Build history of the part. All positions in model axes, mm. A direction names the side the tool comes from. Round coordinates to 2 decimals unless told otherwise and drop trailing zeros. Loops run counter-clockwise (first coordinate to the right, second up) from the corner with the lowest first, then second, coordinate; pieces in that order, holes last. Notation, with made-up numbers: (-16, -20) -> (-4, -20) arc R21 ccw to (-4, -13) -> close; hole circle Ø7 at (20, 81). An arc over 180 degrees is marked (long way). Put each result on its own line as item: value. Start each with the question number.
```python
from build123d import *

# Parameters (mm, degrees)
SKETCH1_R           = 36.125
BOSS_EXTRUDE1_DEPTH = 12
SKETCH3_R           = 37.625
BOSS_EXTRUDE3_DEPTH = 1.5
SKETCH4_R           = 37.625
BOSS_EXTRUDE4_DEPTH = 1.5
SKETCH5_R           = 28
BOSS_EXTRUDE5_DEPTH = 10
SKETCH6_R           = 12.5
CUT_EXTRUDE1_DEPTH  = 25


with BuildPart() as part:
    # Sketch1 → Boss-Extrude1 (new body)
    with BuildSketch(Plane(origin=(0, 0, 0), x_dir=(1, 0, 0), z_dir=(0, 1, 0))):
        Circle(SKETCH1_R)
    extrude(amount=BOSS_EXTRUDE1_DEPTH)

    # Sketch3 → Boss-Extrude3 (add)
    with BuildSketch(Plane(origin=(0, 12, 0), x_dir=(1, 0, 0), z_dir=(0, 1, 0))):
        Circle(SKETCH3_R)
    extrude(amount=BOSS_EXTRUDE3_DEPTH)

    # Sketch4 → Boss-Extrude4 (add)
    with BuildSketch(Plane.XZ):
        Circle(SKETCH4_R)
    extrude(amount=BOSS_EXTRUDE4_DEPTH)

    # Sketch5 → Boss-Extrude5 (add)
    with BuildSketch(Plane.XZ.offset(1.5)):
        Circle(SKETCH5_R)
    extrude(amount=BOSS_EXTRUDE5_DEPTH)

    # Sketch6 → Cut-Extrude1 (cut)
    with BuildSketch(Plane(origin=(0, 13.5, 0), x_dir=(1, 0, 0), z_dir=(0, 1, 0))):
        Circle(SKETCH6_R)
    extrude(amount=-CUT_EXTRUDE1_DEPTH, mode=Mode.SUBTRACT)


solid = part.part
```
Item 1: 3-axis set-ups, long thin cutter, end or side, ignore diameter. For faces 4 (the face through (6, -11.5, -12)), 5 (the face through (-28, -1.5, -3)), 6 (the face through (-34, 0, 14)): which of +Z, -Z, +X, -X, +Y, -Y reach the whole face in a straight line?
Item 2: Cut at B-B on x = 0. Write the cut outline in (y, z) (3 decimals).
Item 3: Pull direction Y, two halves, no side cores. Call faces 1 (the face through (19.42, 5.92, -30.46)), 2 (the face through (-9, 13.5, -9)), 3 (the face through (-27.73, 12.74, -25.43)): +Y half, -Y half, draft (parallel to the pull), parting line (faces both ways), or undercut.
Item 4: Cut at D-D on y = -5.25. Write the cut outline in (x, z), then the cut area to 3 significant figures.
Item 5: Drop flat-ended pins along their axis: pin 1 (10 mm diameter, centred on y = 8.5, z = 1.5, fed in from -X) (3 decimals); pin 2 (5 mm diameter, centred on y = 4.5, z = 22, fed in from +X); pin 3 (5 mm diameter, centred on x = -8, y = -0.5, fed in from +Z); pin 4 (10 mm diameter, centred on x = 29, z = 21, fed in from -Y). Give the stop position or say it passes through.
Item 6: Wall check: line 1 (Z direction, x = 0, y = 2) (3 decimals); line 2 (Y direction, x = 32.5, z = -18). Give the ranges that are in metal, low to high. Write a range as from..to.
Item 7: Cut at C-C on z = -33. Write the cut outline in (x, y), then the cut area to 3 significant figures.
Item 8: Cut at A-A on z = 0. Write the cut outline in (x, y) (3 decimals), then the cut area to 3 significant figures.
Ans:
1. face 4: +Z, -Z, +X, -X, -Y
1. face 5: -Y
1. face 6: none
2. outline: (-11.5, -28) -> (-1.5, -28) -> (-1.5, -37.625) -> (0, -37.625) -> (0, -36.125) -> (12, -36.125) -> (12, -37.625) -> (13.5, -37.625) -> (13.5, -12.5) -> (-11.5, -12.5) -> close; (-11.5, 12.5) -> (13.5, 12.5) -> (13.5, 37.625) -> (12, 37.625) -> (12, 36.125) -> (0, 36.125) -> (0, 37.625) -> (-1.5, 37.625) -> (-1.5, 28) -> (-11.5, 28) -> close
3. face 1: undercut
3. face 2: +Y half
3. face 3: draft
4. outline: circle Ø56 at (0, 0); hole circle Ø25 at (0, 0)
4. area: 1,970 mm2
5. pin 1: stops at x = -37.625
5. pin 2: stops at x = 30.41
5. pin 3: stops at z = 37.22
5. pin 4: stops at y = -1.5
6. line 1: z = -36.125..-12.5, 12.5..36.125
6. line 2: y = -1.5..0, 12..13.5
7. outline: (-18.07, -1.5) -> (18.07, -1.5) -> (18.07, 0) -> (14.7, 0) -> (14.7, 12) -> (18.07, 12) -> (18.07, 13.5) -> (-18.07, 13.5) -> (-18.07, 12) -> (-14.7, 12) -> (-14.7, 0) -> (-18.07, 0) -> close
7. area: 461 mm2
8. outline: (-37.625, -1.5) -> (-28, -1.5) -> (-28, -11.5) -> (-12.5, -11.5) -> (-12.5, 13.5) -> (-37.625, 13.5) -> (-37.625, 12) -> (-36.125, 12) -> (-36.125, 0) -> (-37.625, 0) -> close; (12.5, -11.5) -> (28, -11.5) -> (28, -1.5) -> (37.625, -1.5) -> (37.625, 0) -> (36.125, 0) -> (36.125, 12) -> (37.625, 12) -> (37.625, 13.5) -> (12.5, 13.5) -> close
8. area: 1,030 mm2
